Geometry: final body of the model. Coordinates: model frame, mm. Face numbers are marked on the shaded views. A direction names the side the tool comes from. Coordinates: 2 decimals unless noted, no trailing zeros. Order: outer loops, then holes, each group sorted by start corner. A loop starts at its lowest first (then second) coordinate and runs counter-clockwise, first axis right, second up. Notation, with made-up numbers: M -32.5,51 L 2.5,51 A7 ccw 2.5,59 Z; hole C 36,12.25 d3. An arc over 180 degrees is marked long. Write item = value, one per line. Start each with the question number.
```python
from build123d import *

# Parameters (mm, degrees)
BOSS_EXTRU_1_DEPTH      = 30
ENL_V_MAT_EXTRU_1_DEPTH = 13


with BuildPart() as part:
    # Esquisse2 → Boss.-Extru.1 (new body)
    with BuildSketch(Plane.XY):
        Polygon((0, 0), (-39.274217667, 0), (-39.274217667, 12), (10.725782333, 12), (10.725782333, 9), (7.150521556, 9), (7.150521556, 6), (3.575260778, 6), (3.575260778, 3), (0, 3), align=None)
    extrude(amount=BOSS_EXTRU_1_DEPTH)

    # Esquisse3 → Enlèv. mat.-Extru.1 (cut, through all)
    with BuildSketch(Plane.XZ):
        with BuildLine():
            Line((-9.274217667, 10), (-39.274217667, 10))
            Line((-39.274217667, 10), (-39.274217667, 20))
            Line((-39.274217667, 20), (-9.274217667, 20))
            ThreePointArc((-9.274217667, 20), (-4.274217667, 15), (-9.274217667, 10))
        make_face()
    extrude(amount=-ENL_V_MAT_EXTRU_1_DEPTH, mode=Mode.SUBTRACT)


solid = part.part
```
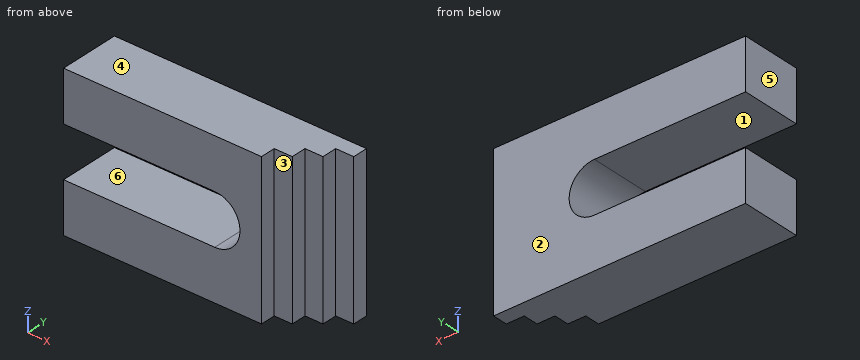
Item 1: First-contact query: pin 1 (3.5 mm diameter, centred on y = 4.5, z = 19.5, fed in from +X); pin 2 (4 mm diameter, centred on x = 9, z = 19.5, fed in from -Y); pin 3 (3.5 mm diameter, centred on y = 1, z = 15, fed in from +X); pin 4 (1 mm diameter, centred on x = -11.5, y = 1.5, fed in from -Z). Flat tips, straight axial feed; report the tip coordinate or a pass-through.
Item 2: Material intervals for probe 1 along Z at (x, y) = (-27.5, 6.5); probe 2 along X at (y, z) = (5.25, 4); probe 3 along X at (y, z) = (7.5, 6.75), sorted ascending. Write a range as [from, to].
Item 3: Section query A-A on x = -13.5. Output: boundary loops of the cut face in (y, z), and give its area (3 significant figures).
Item 4: Section query D-D on y = 2.5. Output: boundary loops of the cut face in (x, z).
Item 5: Section query B-B on y = 7.5. Output: boundary loops of the cut face in (x, z).
Item 6: Draft query along Z for the marked faces 4, 5 and 6. Return one class per face: pulls with the +Z half, pulls with the -Z half, needs draft (parallel to the pull), parting line crosses it, or undercut.
Item 7: Section query C-C on z = 20.75. Output: boundary loops of the cut face in (x, y), and give its area (3 significant figures).
Item 8: Reachability of the marked faces 1, 2 and 3 from +Z, -Z, +X, -X, +Y, -Y: full face, straight path, thin tool, end or side. Return the list, or none.
Ans:
q1.pin_1 = 7.15
q1.pin_2 = 6
q1.pin_3 = 0
q1.pin_4 = 0
q2.probe_1 = [0, 10], [20, 30]
q2.probe_2 = [-39.27, 3.58]
q2.probe_3 = [-39.27, 7.15]
q3.outline = M 0,0 L 12,0 L 12,10 L 0,10 Z; M 0,20 L 12,20 L 12,30 L 0,30 Z
q3.area = 240 mm^2
q4.outline = M -39.27,0 L 0,0 L 0,30 L -39.27,30 L -39.27,20 L -9.27,20 A5 cw -9.27,10 L -39.27,10 Z
q5.outline = M -39.27,0 L 7.15,0 L 7.15,30 L -39.27,30 L -39.27,20 L -9.27,20 A5 cw -9.27,10 L -39.27,10 Z
q6.face_4 = pulls with the +Z half
q6.face_5 = needs draft
q6.face_6 = undercut
q7.outline = M -39.27,0 L 0,0 L 0,3 L 3.58,3 L 3.58,6 L 7.15,6 L 7.15,9 L 10.73,9 L 10.73,12 L -39.27,12 Z
q7.area = 536 mm^2
q8.face_1 = -X, +Y, -Y
q8.face_2 = +Z, -Z, +X, -X, +Y
q8.face_3 = +Z, -Z, +X, -Y
